Could you check a few things on this model? Use its own coordinates, in mm. Coordinates: 2 decimals unless noted, no trailing zeros. Loops run counter-clockwise (first coordinate to the right, second up) from the corner with the lowest first, then second, coordinate; pieces in that order, holes last. Notation, with made-up numbers: (10, 58) - (23, 58) arc R5 ccw to (23, 63) - close; hole circle Ø6 at (-19.75, 87.5). An arc over 180 degrees is marked (long way). One line per item, written item: value. Start each with the question number.
(1) I'm going to push flat-ended pins straight in: P1, Ø10, axis at x = -224.5, y = 12.5, coming from the +Z side; P2, Ø12, axis at y = 1, z = -118, coming from the +X side; P3, Ø1.5, axis at x = 65.5, z = -280.5, coming from the +Y side. Where does each tip first touch, or does it pass through?
(2) If we mould it in two halves opening along X, with no side actions, what happens to faces 1 (the face through (-113.359, -1.521, -174.565)), 2 (the face through (-6, 0, 97))? For each: pulls with the +X half, pulls with the -X half, needs draft (parallel to the pull), parting line crosses it, or undercut.
(3) If we section it at C-C on z = -115.5: Write out the boundary of the cut face in (x, y), then the cut area to 3 significant figures.
(4) If we section it at A-A on x = 288: Write out the boundary of the cut face in (y, z).
(5) If I drill on line 1 along Z through (x, y) = (98.5, -0.8); line 2 along X through (y, z) = (-0.75, -365.4); line 3 along X through (y, z) = (-1.7, -70.35), over which ranges is the centre line in solid material (lowest first)? Write a range as from..to.
(6) If we section it at B-B on x = 14.5: Write out the boundary of the cut face in (y, z).
```python
from build123d import *

# Parameters (mm, degrees)
SKETCH1_W                    = 856
SKETCH1_H                    = 798
BASE_FLANGE1_DEPTH           = 3
SKETCH8_R                    = 60
CUT_EXTRUDE1_DEPTH           = 3
M4_CLEARANCE_HOLE1_D         = 4.5
CIRPATTERN1_COUNT            = 6
EDGE_FLANGE1_STRIP_W         = 18
EDGE_FLANGE1_STRIP_H         = 3
EDGE_FLANGE1_STRIP_CUT_DEPTH = 856
EDGE_FLANGE1_DEPTH           = 856
M5_CLEARANCE_HOLE3_D         = 5.5
M5_CLEARANCE_HOLE4_D         = 5.5
LPATTERN1_COUNT              = 5
LPATTERN1_PITCH              = 204
F_7_1_7_1_DIAMETER_HOLE1_D   = 7.1
LPATTERN2_COUNT              = 5
LPATTERN2_PITCH              = 204
SKETCH26_R                   = 15
CUT_EXTRUDE2_DEPTH           = 3
M5_CLEARANCE_HOLE6_D         = 5.5
FILLET1_R                    = 5
FILLET2_R                    = 10
SKETCH29_R                   = 15
CUT_EXTRUDE3_DEPTH           = 10
M5_CLEARANCE_HOLE7_D         = 5.5
CIRPATTERN2_COUNT            = 3
M6_CLEARANCE_HOLE1_D         = 6.6


# Sheet-metal steps are written as plain solids
with BuildPart() as part:
    # Sketch1 → Base-Flange1 (new body)
    with BuildSketch(Plane(origin=(0, 0, 0), x_dir=(1, 0, 0), z_dir=(0, 1, 0))):
        with Locations((0, -11.5)):
            Rectangle(SKETCH1_W, SKETCH1_H)
    extrude(amount=-BASE_FLANGE1_DEPTH)

    # Sketch8 → Cut-Extrude1 (cut)
    with BuildSketch(Plane(origin=(0, 0, 0), x_dir=(1, 0, 0), z_dir=(0, 1, 0))):
        with Locations(Location((0, 0, 0), (0, 0, 270))):
            Circle(SKETCH8_R)
    extrude(amount=-CUT_EXTRUDE1_DEPTH, mode=Mode.SUBTRACT)

    # M4 Clearance Hole1 (through all)
    with Locations(Plane(origin=(0, -3, 0), x_dir=(-1, 0, 0), z_dir=(0, -1, 0))):
        with Locations((56.724663948, 32.75)):
            m4_clearance_hole1 = Hole(M4_CLEARANCE_HOLE1_D / 2)

    # CirPattern1: M4 Clearance Hole1 ×6 about axis
    cirpattern1_axis = Axis((0, 0, 0), (0, 1, 0))
    for i in range(1, CIRPATTERN1_COUNT):
        add(m4_clearance_hole1.rotate(cirpattern1_axis, i * 360 / CIRPATTERN1_COUNT), mode=Mode.SUBTRACT)

    # Edge-Flange1 strip (across the edge) → Edge-Flange1 strip cut (cut)
    with BuildSketch(Plane(origin=(428, 0, -387.5), x_dir=(0, 0, 1), z_dir=(-1, 0, 0))):
        with Locations((-3, -1.5)):
            Rectangle(EDGE_FLANGE1_STRIP_W, EDGE_FLANGE1_STRIP_H)
    extrude(amount=EDGE_FLANGE1_STRIP_CUT_DEPTH, mode=Mode.SUBTRACT)

    # Edge-Flange1 section (across the edge) → Edge-Flange1 (add)
    with BuildSketch(Plane(origin=(428, 0, -387.5), x_dir=(0, 0, 1), z_dir=(-1, 0, 0))):
        with BuildLine():
            Line((0, 3), (0, 20))
            Line((0, 20), (3, 20))
            Line((3, 20), (3, 3))
            ThreePointArc((3, 3), (3.878679656, 0.878679656), (6, 0))
            Line((6, 0), (6, -3))
            ThreePointArc((6, -3), (1.757359313, -1.242640687), (0, 3))
        make_face()
    extrude(amount=EDGE_FLANGE1_DEPTH)

    # M5 Clearance Hole3 (through all)
    with Locations(Plane(origin=(0, -3, 0), x_dir=(-1, 0, 0), z_dir=(0, -1, 0))):
        with Locations((419, 365.4), (419, 182.7), (419, 0), (419, -182.7), (419, -365.4)):
            m5_clearance_hole3 = Hole(M5_CLEARANCE_HOLE3_D / 2)

    # Mirror2: M5 Clearance Hole3 across plane
    add(m5_clearance_hole3.mirror(Plane(origin=(0, 0, 0), x_dir=(0, 0, 1), z_dir=(1, 0, 0))), mode=Mode.SUBTRACT)

    # M5 Clearance Hole4 (through all)
    with Locations(Plane(origin=(0, 0, 0), x_dir=(1, 0, 0), z_dir=(0, 1, 0))):
        with Locations((-408, -400.5)):
            m5_clearance_hole4 = Hole(M5_CLEARANCE_HOLE4_D / 2)

    # LPattern1: M5 Clearance Hole4 ×5
    with Locations(*[(i * LPATTERN1_PITCH, 0, 0) for i in range(1, LPATTERN1_COUNT)]):
        add(m5_clearance_hole4, mode=Mode.SUBTRACT)

    # Ø7.1 (7.1) Diameter Hole1 (through all)
    with Locations(Plane.XY.offset(-384.5)):
        with Locations((-408, 11)):
            f_7_1_7_1_diameter_hole1 = Hole(F_7_1_7_1_DIAMETER_HOLE1_D / 2)

    # LPattern2: Ø7.1 (7.1) Diameter Hole1 ×5
    with Locations(*[(i * LPATTERN2_PITCH, 0, 0) for i in range(1, LPATTERN2_COUNT)]):
        add(f_7_1_7_1_diameter_hole1, mode=Mode.SUBTRACT)

    # Sketch26 → Cut-Extrude2 (cut)
    with BuildSketch(Plane(origin=(0, -3, 0), x_dir=(-1, 0, 0), z_dir=(0, -1, 0))):
        with Locations(Location((126.0075, 166.500832071, 0), (0, 0, 90))):
            Circle(SKETCH26_R)
    extrude(amount=-CUT_EXTRUDE2_DEPTH, mode=Mode.SUBTRACT)

    # M5 Clearance Hole6 (through all)
    with Locations(Plane(origin=(0, -3, 0), x_dir=(-1, 0, 0), z_dir=(0, -1, 0))):
        with Locations((148.87057066, 179.700832071), (126.0075, 140.100832071), (103.14442934, 179.700832071)):
            Hole(M5_CLEARANCE_HOLE6_D / 2)

    # Fillet1
    fillet1_edges = [part.edges().sort_by_distance(p)[0] for p in [
        (428, -1.5, 410.5),
        (-428, -1.5, 410.5),
    ]]
    fillet(fillet1_edges, radius=FILLET1_R)

    # Fillet2
    fillet2_edges = [part.edges().sort_by_distance(p)[0] for p in [
        (428, 20, -386),
        (-428, 20, -386),
    ]]
    fillet(fillet2_edges, radius=FILLET2_R)

    # Sketch29 → Cut-Extrude3 (cut)
    with BuildSketch(Plane(origin=(0, 0, 0), x_dir=(1, 0, 0), z_dir=(0, 1, 0))):
        with Locations(Location((126, 250.500832071, 0), (0, 0, 270))):
            Circle(SKETCH29_R)
    extrude(amount=-CUT_EXTRUDE3_DEPTH, mode=Mode.SUBTRACT)

    # M5 Clearance Hole7 (through all)
    with Locations(Plane(origin=(0, 0, 0), x_dir=(1, 0, 0), z_dir=(0, 1, 0))):
        with Locations((126, 224.000832071)):
            m5_clearance_hole7 = Hole(M5_CLEARANCE_HOLE7_D / 2)

    # CirPattern2: M5 Clearance Hole7 ×3 about axis
    cirpattern2_axis = Axis((126, 0, -250.500832071), (0, 1, 0))
    for i in range(1, CIRPATTERN2_COUNT):
        add(m5_clearance_hole7.rotate(cirpattern2_axis, i * 360 / CIRPATTERN2_COUNT), mode=Mode.SUBTRACT)

    # M6 Clearance Hole1 (through all)
    with Locations(Plane(origin=(0, 0, 0), x_dir=(1, 0, 0), z_dir=(0, 1, 0))):
        with Locations((98.5, -44.65), (168.5, -44.65), (168.5, 70.35), (98.5, 70.35)):
            Hole(M6_CLEARANCE_HOLE1_D / 2)


solid = part.part
```
Values:
1. P1: stops at z = -384.5
1. P2: stops at x = 428
1. P3: stops at y = 0
2. face 1: undercut
2. face 2: needs draft
3. outline: (-428, -3) - (428, -3) - (428, 0) - (-428, 0) - close
3. area: 2,570 mm2
4. outline: (-3, -381.5) arc R6 ccw to (3, -387.5) - (20, -387.5) - (20, -384.5) - (3, -384.5) arc R3 cw to (0, -381.5) - (0, 410.5) - (-3, 410.5) - close
5. line 1: z = -386.14..-73.65, -67.05..41.35, 47.95..410.5
5. line 2: x = -428..-421.75, -416.25..416.25, 421.75..428
5. line 3: x = -428..95.2, 101.8..165.2, 171.8..428
6. outline: (-3, -381.5) arc R6 ccw to (3, -387.5) - (20, -387.5) - (20, -384.5) - (3, -384.5) arc R3 cw to (0, -381.5) - (0, -58.22) - (-3, -58.22) - close; (-3, 58.22) - (0, 58.22) - (0, 410.5) - (-3, 410.5) - close
